Can you work these out from the model? Positions are in its coordinate system, mm. A direction names the side the tool comes from. Give positions to 0.01 mm unless a question says otherwise; leave off trailing zeros. Order: outer loops, then holes, each group sorted by start corner. A loop starts at its lowest first (then second) coordinate and runs counter-clockwise, first axis right, second up. Notation, with made-up numbers: (39.5, 8.5) - (47.5, 8.5) arc R19 cw to (47.5, 12.5) - close; hole circle Ø1 at (-30.5, -26). An arc over 180 degrees is marked (long way). Use one line per item in the form item = value. Start each with the question number.
1) Which directions (+Z, -Z, +X, -X, +Y, -Y) give clear straight access to the entire face, cutting with the end or side of a thin tool? Please do faces 1 (the flat face through (1535, 5, -499.745)), 2 (the flat face through (725, -422.275, -451)).
2) Please list where these lines run through material, in increasing order: probe 1 along X at (y, z) = (-358, 121.5); probe 2 along Z at (x, y) = (242, 362.5) (3 decimals).
3) Suppose I cut it at B-B, the plane x = 855.5. Write out the boundary of the cut face in (y, z) (3 decimals), and give its area (3 significant figures).
4) Suppose I cut it at A-A, the plane z = 215. Write out the boundary of the cut face in (x, y) (3 decimals).
5) We'd pull the mould along Y, two halves only. Please class faces 3 (the flat face through (725, 422.275, -451)), 4 (the flat face through (40, 5, -499.745)), 5 (the flat face through (725, -373, -504.825)): released by +Y, released by -Y, zero draft, split by the parting line, or undercut.
```python
from build123d import *

# Parameters (mm, degrees)
BOSS_EXTRUDE1_DEPTH   = 1574.8
BOSS_EXTRUDE1_2_DEPTH = 1574.8
BOSS_EXTRUDE1_3_DEPTH = 1574.8
BOSS_EXTRUDE1_4_DEPTH = 1574.8
BOSS_EXTRUDE2_START   = -498.751917
BOSS_EXTRUDE2_DEPTH   = 997.503834
BOSS_EXTRUDE3_REACH   = 846.55


with BuildPart() as part:
    # Sketch2 → Boss-Extrude1 (new body)
    with BuildSketch(Plane(origin=(0, 0, 0), x_dir=(0, 0, -1), z_dir=(1, 0, 0))):
        Polygon((-504.825, -346.075), (-504.825, -422.275), (-428.625, -422.275), (-428.625, -417.195), (-498.751917293, -417.195), (-498.751917293, -346.075), align=None)
    extrude(amount=BOSS_EXTRUDE1_DEPTH)



with BuildPart() as body_2:
    # Sketch2 → Boss-Extrude1 2 (new body)
    with BuildSketch(Plane(origin=(0, 0, 0), x_dir=(0, 0, -1), z_dir=(1, 0, 0))):
        Polygon((498.751917293, -417.195), (498.751917293, -346.075), (504.825, -346.075), (504.825, -422.275), (428.625, -422.275), (428.625, -417.195), align=None)
    extrude(amount=BOSS_EXTRUDE1_2_DEPTH)


with BuildPart() as body_3:
    # Sketch2 → Boss-Extrude1 3 (new body)
    with BuildSketch(Plane(origin=(0, 0, 0), x_dir=(0, 0, -1), z_dir=(1, 0, 0))):
        Polygon((428.625, 417.195), (498.751917293, 417.195), (498.751917293, 346.075), (504.825, 346.075), (504.825, 422.275), (428.625, 422.275), align=None)
    extrude(amount=BOSS_EXTRUDE1_3_DEPTH)


with BuildPart() as body_4:
    # Sketch2 → Boss-Extrude1 4 (new body)
    with BuildSketch(Plane(origin=(0, 0, 0), x_dir=(0, 0, -1), z_dir=(1, 0, 0))):
        Polygon((-498.751917293, 417.195), (-498.751917293, 346.075), (-504.825, 346.075), (-504.825, 422.275), (-428.625, 422.275), (-428.625, 417.195), align=None)
    extrude(amount=BOSS_EXTRUDE1_4_DEPTH)


with BuildPart() as part_1:
    add(part.part)

    add(body_2.part)  # Boss-Extrude2 merges body 2

    add(body_3.part)  # Boss-Extrude2 merges body 3

    add(body_4.part)  # Boss-Extrude2 merges body 4
    # Sketch3 → Boss-Extrude2 (add)
    with BuildSketch(Plane.XY.offset(BOSS_EXTRUDE2_START)):
        Polygon((0, -422.275), (0, -346.075), (5.08, -346.075), (5.08, -417.195), (76.2, -417.195), (76.2, -422.275), align=None)
        Polygon((76.2, 422.275), (0, 422.275), (0, 346.075), (5.08, 346.075), (5.08, 417.195), (76.2, 417.195), align=None)
        Polygon((1574.8, 422.275), (1574.8, 346.075), (1569.72, 346.075), (1569.72, 417.195), (1498.6, 417.195), (1498.6, 422.275), align=None)
        Polygon((1498.6, -422.275), (1574.8, -422.275), (1574.8, -346.075), (1569.72, -346.075), (1569.72, -417.195), (1498.6, -417.195), align=None)
    extrude(amount=BOSS_EXTRUDE2_DEPTH)

    # Sketch4 → Boss-Extrude3 (add, up to next)
    with BuildSketch(Plane(origin=(0, 422.275, 0), x_dir=(1, 0, 0), z_dir=(0, 1, 0)), mode=Mode.PRIVATE) as boss_extrude3_sk1:
        Polygon((0, 504.825), (0, 428.625), (5.08, 428.625), (5.08, 499.745), (76.2, 499.745), (76.2, 504.825), align=None)
    boss_extrude3_tool1 = extrude(boss_extrude3_sk1.sketch, amount=-BOSS_EXTRUDE3_REACH, mode=Mode.PRIVATE) - part_1.part
    add(boss_extrude3_tool1.solids().sort_by_distance((1.077631, 422.275, -466.725))[0])
    # Sketch4 → Boss-Extrude3 (add, up to next)
    with BuildSketch(Plane(origin=(0, 422.275, 0), x_dir=(1, 0, 0), z_dir=(0, 1, 0)), mode=Mode.PRIVATE) as boss_extrude3_sk2:
        Polygon((76.2, -504.825), (0, -504.825), (0, -428.625), (5.08, -428.625), (5.08, -499.745), (76.2, -499.745), align=None)
    boss_extrude3_tool2 = extrude(boss_extrude3_sk2.sketch, amount=-BOSS_EXTRUDE3_REACH, mode=Mode.PRIVATE) - part_1.part
    add(boss_extrude3_tool2.solids().sort_by_distance((38.1, 422.275, 503.747369))[0])
    # Sketch4 → Boss-Extrude3 (add, up to next)
    with BuildSketch(Plane(origin=(0, 422.275, 0), x_dir=(1, 0, 0), z_dir=(0, 1, 0)), mode=Mode.PRIVATE) as boss_extrude3_sk3:
        Polygon((1574.8, -504.825), (1574.8, -428.625), (1569.72, -428.625), (1569.72, -499.745), (1498.6, -499.745), (1498.6, -504.825), align=None)
    boss_extrude3_tool3 = extrude(boss_extrude3_sk3.sketch, amount=-BOSS_EXTRUDE3_REACH, mode=Mode.PRIVATE) - part_1.part
    add(boss_extrude3_tool3.solids().sort_by_distance((1573.722369, 422.275, 466.725))[0])
    # Sketch4 → Boss-Extrude3 (add, up to next)
    with BuildSketch(Plane(origin=(0, 422.275, 0), x_dir=(1, 0, 0), z_dir=(0, 1, 0)), mode=Mode.PRIVATE) as boss_extrude3_sk4:
        Polygon((1498.6, 504.825), (1574.8, 504.825), (1574.8, 428.625), (1569.72, 428.625), (1569.72, 499.745), (1498.6, 499.745), align=None)
    boss_extrude3_tool4 = extrude(boss_extrude3_sk4.sketch, amount=-BOSS_EXTRUDE3_REACH, mode=Mode.PRIVATE) - part_1.part
    add(boss_extrude3_tool4.solids().sort_by_distance((1536.7, 422.275, -503.747369))[0])


solid = part_1.part
```
Result sheet:
q1.face_1 = none
q1.face_2 = +Z, -Z, +X, -X, -Y
q2.probe_1 = 0 to 5.08, 1569.72 to 1574.8
q2.probe_2 = -504.825 to -498.752, 498.752 to 504.825
q3.outline = (-422.275, -504.825) - (-346.075, -504.825) - (-346.075, -498.752) - (-417.195, -498.752) - (-417.195, -428.625) - (-422.275, -428.625) - close; (-422.275, 428.625) - (-417.195, 428.625) - (-417.195, 498.752) - (-346.075, 498.752) - (-346.075, 504.825) - (-422.275, 504.825) - close; (346.075, -504.825) - (422.275, -504.825) - (422.275, -428.625) - (417.195, -428.625) - (417.195, -498.752) - (346.075, -498.752) - close; (346.075, 498.752) - (417.195, 498.752) - (417.195, 428.625) - (422.275, 428.625) - (422.275, 504.825) - (346.075, 504.825) - close
q3.area = 3,280 mm²
q4.outline = (0, -422.275) - (76.2, -422.275) - (76.2, -417.195) - (5.08, -417.195) - (5.08, -346.075) - (0, -346.075) - close; (0, 346.075) - (5.08, 346.075) - (5.08, 417.195) - (76.2, 417.195) - (76.2, 422.275) - (0, 422.275) - close; (1498.6, -422.275) - (1574.8, -422.275) - (1574.8, -346.075) - (1569.72, -346.075) - (1569.72, -417.195) - (1498.6, -417.195) - close; (1498.6, 417.195) - (1569.72, 417.195) - (1569.72, 346.075) - (1574.8, 346.075) - (1574.8, 422.275) - (1498.6, 422.275) - close
q5.face_3 = released by +Y
q5.face_4 = undercut
q5.face_5 = zero draft
